The model under review builds one solid part; all positions refer to its coordinate system, in mm. Round coordinates to 2 decimals unless told otherwise and drop trailing zeros. Order: outer loops, then holes, each group sorted by start corner. A loop starts at its lowest first (then second) coordinate and runs counter-clockwise, first axis right, second up.
1) Consider section A-A (z = -60). Give the boundary of the cut face in (x, y), then the cut area to 3 significant figures.
2) Clearance check with a flat-ended pin moving along its axis: P1, Ø4, axis at x = -57.06, z = -18.54, coming from the +Y side. State where the tip first meets the part, or that it passes through.
3) Consider section C-C (x = -28). Give the boundary of the cut face in (y, z).
4) To check wall thickness, follow L1, parallel to X at y = 2.5, z = 49; L2, parallel to X at y = 0.75, z = -20; L3, parallel to X at y = 2.6, z = 46. State the ranges of each line that lie inside material, in increasing order.
5) Consider section B-B (y = 1.35). Give the number of separate pieces and of enclosed holes in the cut face, then the cut area to 3 significant figures.
6) Consider section D-D (z = -2). Give the boundary of the cut face in (x, y), then the cut area to 3 significant figures.
7) Mouldability with a two-part tool opening along X and no side actions: class faces 1 (the face through (-1, 3, -7)), 2 (the face through (41.819, 1.479, 57.656)), 3 (the face through (-34.83, 1.48, -48.86)), 4 (the face through (-60.56, 1.48, -18.69)) as pulls with the +X half, pulls with the -X half, needs draft (parallel to the pull), parting line crosses it, or undercut.
from build123d import *

# Parameters (mm, degrees)
ESQUISSE2_R        = 3.5
ESQUISSE2_R_2      = 1
BOSS_EXTRU_1_DEPTH = 3
CHANFREIN1_SIZE    = 5


with BuildPart() as part:
    # Esquisse2 → Boss.-Extru.1 (new body)
    with BuildSketch(Plane(origin=(0, 0, 0), x_dir=(1, 0, 0), z_dir=(0, 1, 0))):
        Polygon((70.534230275, 22.917960675), (0, 74.16407865), (-70.534230275, 22.917960675), (-43.59255168, -60), (43.59255168, -60), align=None)
        with Locations((-57.063390978, 18.541019662)):
            Circle(ESQUISSE2_R, mode=Mode.SUBTRACT)
        with Locations((0, 60)):
            Circle(ESQUISSE2_R, mode=Mode.SUBTRACT)
        with Locations((57.063390978, 18.541019662)):
            Circle(ESQUISSE2_R, mode=Mode.SUBTRACT)
        with Locations((35.267115138, -48.541019662)):
            Circle(ESQUISSE2_R, mode=Mode.SUBTRACT)
        with Locations((-35.267115138, -48.541019662)):
            Circle(ESQUISSE2_R, mode=Mode.SUBTRACT)
        with Locations((-62.769730075, 20.395121629)):
            Circle(ESQUISSE2_R_2, mode=Mode.SUBTRACT)
        with Locations((-51.35705188, 16.686917696)):
            Circle(ESQUISSE2_R_2, mode=Mode.SUBTRACT)
        with Locations((0, 66)):
            Circle(ESQUISSE2_R_2, mode=Mode.SUBTRACT)
        with Locations((0, 54)):
            Circle(ESQUISSE2_R_2, mode=Mode.SUBTRACT)
        with Locations((62.769730075, 20.395121629)):
            Circle(ESQUISSE2_R_2, mode=Mode.SUBTRACT)
        with Locations((51.35705188, 16.686917696)):
            Circle(ESQUISSE2_R_2, mode=Mode.SUBTRACT)
        with Locations((38.793826651, -53.395121629)):
            Circle(ESQUISSE2_R_2, mode=Mode.SUBTRACT)
        with Locations((31.740403624, -43.686917696)):
            Circle(ESQUISSE2_R_2, mode=Mode.SUBTRACT)
        with Locations((-38.793826651, -53.395121629)):
            Circle(ESQUISSE2_R_2, mode=Mode.SUBTRACT)
        with Locations((-31.740403624, -43.686917696)):
            Circle(ESQUISSE2_R_2, mode=Mode.SUBTRACT)
    extrude(amount=BOSS_EXTRU_1_DEPTH)

    # Chanfrein1
    chanfrein1_edges = [part.edges().sort_by_distance(p)[0] for p in [
        (43.59255168, 1.5, 60),
        (-43.59255168, 1.5, 60),
        (-70.534230275, 1.5, -22.917960675),
        (0, 1.5, -74.16407865),
        (70.534230275, 1.5, -22.917960675),
    ]]
    chamfer(chanfrein1_edges, length=CHANFREIN1_SIZE)


solid = part.part
Answer below:
1. outline: (-19.5, 0) - (-3.5, 0) - (-3.5, 3) - (-19.5, 3) - close; (3.5, 0) - (19.5, 0) - (19.5, 3) - (3.5, 3) - close
1. area: 96.0 mm2
2. P1: passes through
3. outline: (0, -53.82) - (3, -53.82) - (3, 60) - (0, 60) - close
4. L1: x = -47.17 to -38.74, -31.8 to 31.8, 38.74 to 47.17
4. L2: x = -68.39 to -63.69, -61.85 to -60.24, -53.88 to 53.88, 60.24 to 61.85, 63.69 to 68.39
4. L3: x = -48.14 to -37.67, -32.86 to 32.86, 37.67 to 48.14
5. separate pieces: 1
5. enclosed holes: 15
5. area: 12,800 mm2
6. outline: (-63.74, 0) - (63.74, 0) - (63.74, 3) - (-63.74, 3) - close
6. area: 382 mm2
7. face 1: needs draft
7. face 2: pulls with the +X half
7. face 3: pulls with the -X half
7. face 4: undercut
